Here's how the part is built. I have some questions about the finished solid (model axes, mm). A direction names the side the tool comes from. Give positions to 0.01 mm unless a question says otherwise; leave off trailing zeros. Write each loop counter-clockwise with the first axis right and the second up, starting at its lowest first coordinate (ties: lowest second). Pieces come first, ordered by that corner, then holes. Notation, with made-up numbers: (28, 55) -> (51, 55) arc R4 cw to (51, 59) -> close; hole circle Ø8 at (-4.5, 64.25). An arc over 180 degrees is marked (long way). Return JSON: item names as keys, results as strings.
from build123d import *

# Parameters (mm, degrees)
F1_DEPTH = 10


with BuildPart() as f1:
    # F0 (on Front) → F1 (new body)
    with BuildSketch(Plane.XZ):
        with BuildLine():
            Line((-10, 18.563321), (-20, 18.563321))
            Line((-20, 18.563321), (-20, -6.436679))
            Line((-20, -6.436679), (-25, -6.436679))
            Line((-25, -6.436679), (-25, 18.563321))
            Line((-25, 18.563321), (-75, 18.563321))
            ThreePointArc((-75, 18.563321), (-53.033009, -34.469688), (0, -56.436679))
            ThreePointArc((0, -56.436679), (53.033009, -34.469688), (75, 18.563321))
            Line((75, 18.563321), (25, 18.563321))
            Line((25, 18.563321), (25, -6.436679))
            Line((25, -6.436679), (20, -6.436679))
            Line((20, -6.436679), (20, 18.563321))
            Line((20, 18.563321), (10, 18.563321))
            Line((10, 18.563321), (10, -31.436679))
            Line((10, -31.436679), (0, -31.436679))
            Line((0, -31.436679), (-10, -31.436679))
            Line((-10, -31.436679), (-10, 18.563321))
        make_face()
    extrude(amount=F1_DEPTH)


solid = f1.part
1. Suppose I cut it at B-B, the plane y = -6.5. List the corners of the cut face in (x, z) for me.
Taken from the geometry:
{"outline": "(-75, 18.56) arc R75 ccw to (0, -56.44) arc R75 ccw to (75, 18.56) -> (25, 18.56) -> (25, -6.44) -> (20, -6.44) -> (20, 18.56) -> (10, 18.56) -> (10, -31.44) -> (-10, -31.44) -> (-10, 18.56) -> (-20, 18.56) -> (-20, -6.44) -> (-25, -6.44) -> (-25, 18.56) -> close"}
2. Which directions (+Z, -Z, +X, -X, +Y, -Y) give clear straight access to the entire face, cutting with the end or side of a thin tool? Please do faces 1 (the face through (15, -5, 18.563)), 2 (the face through (-22, -5, -6.437)).
Taken from the geometry:
{"face 1": "+Z, +X, -X, +Y, -Y", "face 2": "+Z, +Y, -Y"}
3. If I drill on line 1 (X direction, y = -5, z = 11); line 2 (X direction, y = -7, z = 7); line 3 (X direction, y = -1.75, z = -10.5), over which ranges is the centre line in solid material (lowest first)? Write a range as [from, to].
Taken from the geometry:
{"line 1": "x = [-74.62, -25], [-20, -10], [10, 20], [25, 74.62]", "line 2": "x = [-74.1, -25], [-20, -10], [10, 20], [25, 74.1]", "line 3": "x = [-69.14, -10], [10, 69.14]"}
4. For pin 1 Ø5 at (x, y) = (-4, -3.5) entering from +Z; pin 2 Ø5 at (y, z) = (-6, -16) entering from +X; pin 3 Ø3 at (y, z) = (-3, 11) entering from +X, each with a flat end and sliding along its axis, tell me the tip position at first contact or that it passes through.
Taken from the geometry:
{"pin 1": "stops at z = -31.44", "pin 2": "stops at x = 67.8", "pin 3": "stops at x = 74.75"}
5. Suppose I cut it at D-D, the plane z = 3. List the corners of the cut face in (x, y) for me, and give its area (3 significant figures).
Taken from the geometry:
{"outline": "(-73.37, -10) -> (-25, -10) -> (-25, 0) -> (-73.37, 0) -> close; (-20, -10) -> (-10, -10) -> (-10, 0) -> (-20, 0) -> close; (10, -10) -> (20, -10) -> (20, 0) -> (10, 0) -> close; (25, -10) -> (73.37, -10) -> (73.37, 0) -> (25, 0) -> close", "area": "1,170 mm²"}
6. Suppose I cut it at C-C, the plane z = -20. List the corners of the cut face in (x, y) for me.
Taken from the geometry:
{"outline": "(-64.33, -10) -> (-10, -10) -> (-10, 0) -> (-64.33, 0) -> close; (10, -10) -> (64.33, -10) -> (64.33, 0) -> (10, 0) -> close"}
7. Suppose I cut it at A-A, the plane z = 14. List the corners of the cut face in (x, y) for me, and give its area (3 significant figures).
Taken from the geometry:
{"outline": "(-74.86, -10) -> (-25, -10) -> (-25, 0) -> (-74.86, 0) -> close; (-20, -10) -> (-10, -10) -> (-10, 0) -> (-20, 0) -> close; (10, -10) -> (20, -10) -> (20, 0) -> (10, 0) -> close; (25, -10) -> (74.86, -10) -> (74.86, 0) -> (25, 0) -> close", "area": "1,200 mm²"}
8. If we mould it in two halves opening along X, with no side actions, what happens to faces 3 (the face through (-15, -5, 18.563)), 4 (the face through (-10, -5, -7)), 5 (the face through (20, -5, 6))? For each: released by +X, released by -X, zero draft, split by the parting line, or undercut.
Taken from the geometry:
{"face 3": "zero draft", "face 4": "undercut", "face 5": "undercut"}
